Answer from the drawing. Dimensions are ordinates in mm from the lowest x, y and z of the part. A direction names the side the tool comes from. Coordinates: 2 decimals unless noted, no trailing zeros. Write each loop counter-clockwise with the first axis right and the second up, starting at its lowest first coordinate (ties: lowest second). Pieces come first, ordered by that corner, then holes.
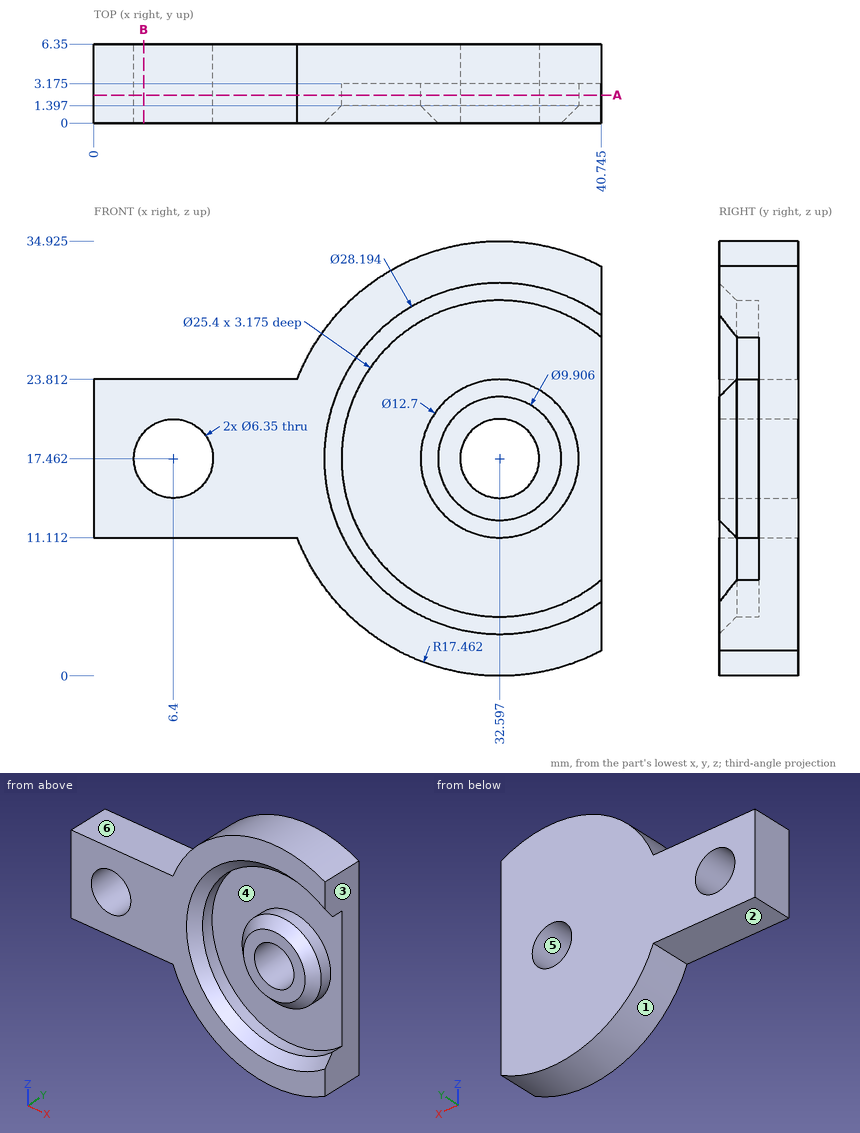
(1) Each of these flat-tipped pins is pushed along its axis until it touches: pin 1 (7.5 mm diameter, centred on x = 32.6, z = 17.46, fed in from +Y); pin 2 (1 mm diameter, centred on x = 7.5, y = 2.5, fed in from -Z); pin 3 (1.5 mm diameter, centred on x = 19, z = 30.5, fed in from +Y). Where does it stop, or does it pass through?
(2) Section B-B, the plane x = 4 is taken. Write down the section's boundary in (y, z).
(3) Find the intervals of material crossed by probe 1 along X at (y, z) = (2.25, 19.5) (1 decimal); probe 2 along Z at (x, y) = (32.5, 4.5) (1 decimal); probe 3 along Z at (x, y) = (12, 4.75), in increasing order.
(4) Which of the six approach directions +Z, -Z, +X, -X, +Y, -Y give full straight-line access (tool end or side, diameter ignored) to the marked faces 1 and 2?
(5) For a pull along Z with two mould halves and no side action, classify the marked faces 3, 4, 5 and 6 as pulls with the +Z half, pulls with the -Z half, needs draft (parallel to the pull), parting line crosses it, or undercut.
(6) Section A-A, the plane y = 2.25 is taken. State how many separate pieces and enclosed holes the cut face has.
Solution:
1. pin 1: stops at y = 6.35
1. pin 2: stops at z = 11.11
1. pin 3: passes through
2. outline: (0, 11.11) - (6.35, 11.11) - (6.35, 15.38) - (0, 15.38) - close; (0, 19.54) - (6.35, 19.54) - (6.35, 23.81) - (0, 23.81) - close
3. probe 1: x = 0 to 4, 8.8 to 20.1, 26.6 to 30.2, 35 to 38.6
3. probe 2: z = 0 to 14.3, 20.6 to 34.9
3. probe 3: z = 11.11 to 23.81
4. face 1: -Z, +Y, -Y
4. face 2: -Z, -X, +Y, -Y
5. face 3: needs draft
5. face 4: undercut
5. face 5: undercut
5. face 6: pulls with the +Z half
6. separate pieces: 2
6. enclosed holes: 2
